Source: CAD feature listing. Evaluate the final solid. Frame: model axes, mm. A direction names the side the tool comes from. Give positions to 0.01 mm unless a question says otherwise; leave off trailing zeros. Loops run counter-clockwise (first coordinate to the right, second up) from the corner with the lowest first, then second, coordinate; pieces in that order, holes last. Notation, with made-up numbers: (79.25, 56) - (89.25, 56) arc R15 cw to (89.25, 70) - close; hole circle Ø8 at (36.25, 61). An arc over 180 degrees is marked (long way). Write each question's results on one line, items separated by ' | '. Start each with the question number.
(1) Cut plane B-B on x = 21.5. Return the cut outline in (y, z) (3 decimals).
(2) Contact query for flat-ended pins moving along their axis: pin 1 (5 mm diameter, centred on x = -147.5, y = -29.5, fed in from -Z); pin 2 (1.9 mm diameter, centred on y = -39, z = 15, fed in from +X) (3 decimals); pin 3 (3 mm diameter, centred on x = -150, y = -30, fed in from +Z). Output: stop coordinate, or through.
(3) Cut plane A-A on y = -28. Return the cut outline in (x, z) (3 decimals).
(4) Pull-direction query (Z, two-part tool) for faces 1 (the flat face through (2, 0, 9)), 2 (the flat face through (2, -59, 12.7)), 3 (the flat face through (-148, -27, 12.7)); classes: pulls with the +Z half, pulls with the -Z half, needs draft (parallel to the pull), parting line crosses it, or undercut.
(5) Reachability of faces 4 (the flat face through (-148, -27, 6.35)), 5 (the flat face through (-142.875, -32, 16)), 6 (the flat face through (142.875, -32, 16)), 7 (the flat face through (148, -27, 6.35)), 8 (the flat face through (2, -59, 6.35)) from +Z, -Z, +X, -X, +Y, -Y: full face, straight path, thin tool, end or side. Return the list, or none.
(6) Cut plane C-C on z = 9.25. Return the cut outline in (x, y) (3 decimals).
(7) Material intervals for line 1 along Z through (x, y) = (-70, -58); line 2 along Y through (x, z) = (-66.5, 9.5) (3 decimals); line 3 along X through (y, z) = (-10, 13) (3 decimals), sorted ascending. Write a range as [from, to].
from build123d import *

# Parameters (mm, degrees)
F0_W     = 63.5
F0_H     = 19.05
F1_DEPTH = 152.4
F2_W     = 9.525
F2_H     = 6.35
F3_DEPTH = 63.501
F4_W     = 9.525
F4_H     = 6.35
F5_DEPTH = 304.801


with BuildPart() as f1:
    # F0 (on Right) → F1 (new body, symmetric)
    with BuildSketch(Plane.YZ):
        with Locations((-31.75, 9.525)):
            Rectangle(F0_W, F0_H)
    extrude(amount=F1_DEPTH, both=True)

    # F2 (on face) → F3 (cut, through all)
    with BuildSketch(Plane.XZ.offset(63.5)):
        with Locations((147.6375, 15.875)):
            Rectangle(F2_W, F2_H)
        with Locations((147.6375, 3.175)):
            Rectangle(F2_W, F2_H)
        with Locations((-147.6375, 15.875)):
            Rectangle(F2_W, F2_H)
        with Locations((-147.6375, 3.175)):
            Rectangle(F2_W, F2_H)
    extrude(amount=-F3_DEPTH, mode=Mode.SUBTRACT)

    # F4 (on face) → F5 (cut, through all)
    with BuildSketch(Plane.YZ.offset(152.4)):
        with Locations((-58.7375, 9.525)):
            Rectangle(F4_W, F4_H)
    extrude(amount=-F5_DEPTH, mode=Mode.SUBTRACT)


solid = f1.part
Ans:
1) outline: (-63.5, 0) - (0, 0) - (0, 19.05) - (-63.5, 19.05) - (-63.5, 12.7) - (-53.975, 12.7) - (-53.975, 6.35) - (-63.5, 6.35) - close
2) pin 1: z = 6.35 | pin 2: x = 142.875 | pin 3: z = 12.7
3) outline: (-152.4, 6.35) - (-142.875, 6.35) - (-142.875, 0) - (142.875, 0) - (142.875, 6.35) - (152.4, 6.35) - (152.4, 12.7) - (142.875, 12.7) - (142.875, 19.05) - (-142.875, 19.05) - (-142.875, 12.7) - (-152.4, 12.7) - close
4) face 1: needs draft | face 2: undercut | face 3: pulls with the +Z half
5) face 4: -Z, -X, +Y, -Y | face 5: +Z, -X, +Y, -Y | face 6: +Z, +X, +Y, -Y | face 7: -Z, +X, +Y, -Y | face 8: +X, -X, -Y
6) outline: (-152.4, -53.975) - (152.4, -53.975) - (152.4, 0) - (-152.4, 0) - close
7) line 1: [0, 6.35], [12.7, 19.05] | line 2: [-53.975, 0] | line 3: [-142.875, 142.875]
